Drawing for the job (mm, zero at the part's lowest x, y, z). Round coordinates to 2 decimals unless told otherwise and drop trailing zeros. Order: outer loops, then holes, each group sorted by start corner. A loop starts at its lowest first (then second) coordinate and runs counter-clockwise, first axis right, second up. Notation, with made-up numbers: (86, 27) -> (94, 27) arc R17 cw to (94, 60) -> close; hole circle Ø10 at (29.25, 58). An arc over 180 degrees is marked (long way). Use CSV: the item, a comma, the result in double quotes.
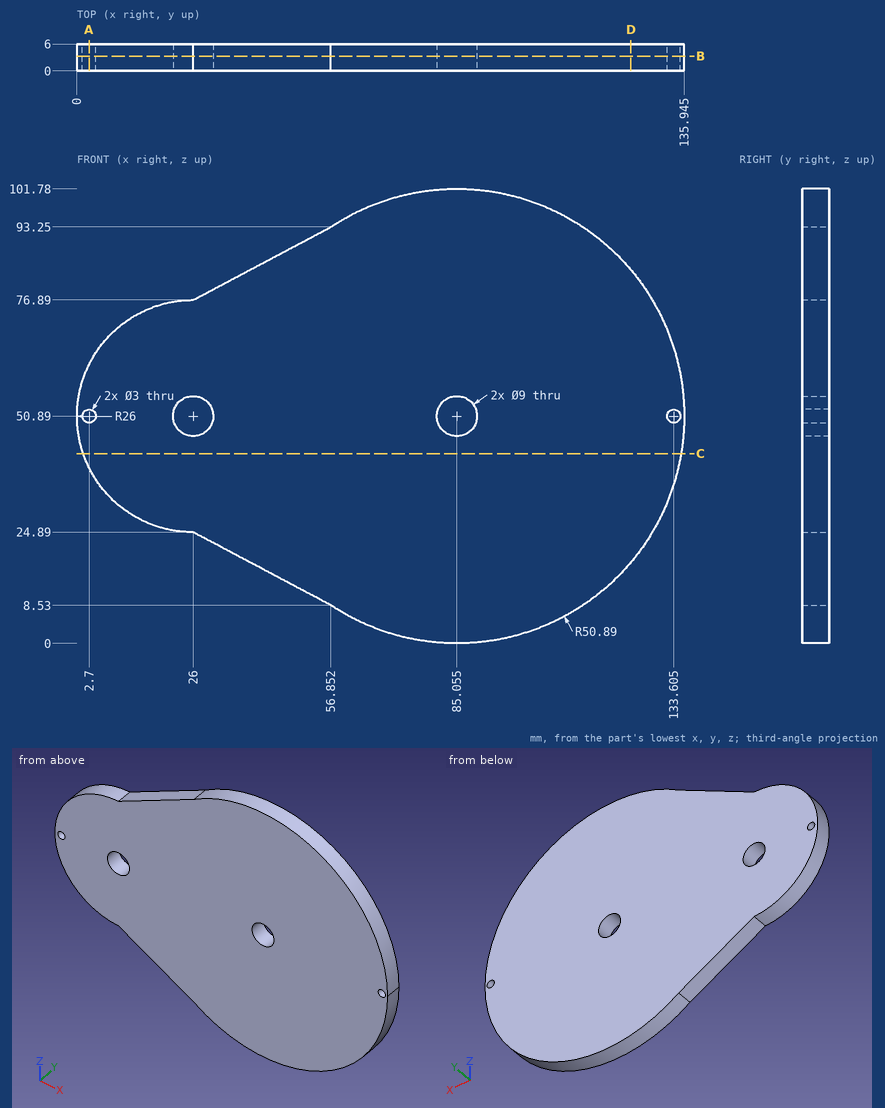
Q1. Probe line 1 along X through (y, z) = (3.15, 52.5); line 2 along Z through (x, y) = (99, 0.4); line 3 along X through (y, z) = (4.45, 61) (1 decimal). List the from-to ranges inside material, lowest first.
From the geometry:
line 1,"x = 0.05 to 21.8, 30.2 to 80.85, 89.26 to 135.92"
line 2,"z = 1.95 to 99.83"
line 3,"x = 2 to 134.9"
Q2. Cut at C-C (z = 42.5). Give the cut face in (x, y).
From the geometry:
outline,"(1.39, 0) -> (135.25, 0) -> (135.25, 6) -> (1.39, 6) -> close"
Q3. Cut at A-A (x = 2.7). Give the cut face in (y, z).
From the geometry:
outline,"(0, 39.35) -> (6, 39.35) -> (6, 49.39) -> (0, 49.39) -> close; (0, 52.39) -> (6, 52.39) -> (6, 62.43) -> (0, 62.43) -> close"
Q4. Pin check, flat tip, straight feed: pin 1 (2 mm diameter, centred on x = 88.5, y = 4, fed in from -Z). Stop position of the tip, or through.
From the geometry:
pin 1,"stops at z = 0.06"
Q5. Cut at D-D (x = 124). Give the cut face in (y, z).
From the geometry:
outline,"(0, 18.13) -> (6, 18.13) -> (6, 83.65) -> (0, 83.65) -> close"
Q6. Cut at B-B (y = 3.3). State how many separate pieces and enclosed holes the cut face has, plus the area to 3 significant figures.
From the geometry:
separate pieces,"1"
enclosed holes,"4"
area,"9,810 mm²"
